Could you check a few things on this drawing? It's one solid part, dimensions in mm from its lowest x, y, z. A direction names the side the tool comes from. Coordinates: 2 decimals unless noted, no trailing zeros. Order: outer loops, then holes, each group sorted by start corner. A loop starts at its lowest first (then second) coordinate and runs counter-clockwise, first axis right, second up. Notation, with made-up numbers: (2.25, -7) - (53.25, -7) arc R18 ccw to (53.25, 6) - close; hole circle Ø10 at (0.5, 0.25). An arc over 180 degrees is marked (long way). Answer in a Markdown table with one row per item. Add a question column.
Item 1: I want a section at C-C (y = 16). Please give me the cut outline in (x, z).
Item 2: Will these pins go through, and if not, where does the flat tip stop? pin 1 Ø12.5 at (x, y) = (27, 18.5) entering from +Z; pin 2 Ø10 at (x, z) = (68, 54) entering from +Y.
Item 3: I want a section at B-B (z = 14). Please give me the cut outline in (x, y).
Item 4: On a 3-axis mill with a long thin cutter (end or side, diameter ignored), from which of +Z, -Z, +X, -X, +Y, -Y can I reach the whole of each face in a straight line? I mean the marked faces 1 and 2. Say none if no direction works.
Item 5: I want a section at A-A (x = 83). Please give me the cut outline in (y, z).
Item 6: If I drill on line 1 along Y through (x, z) = (23.5, 67); line 2 along Z through (x, y) = (48, 1.5), over which ranges is the centre line in solid material (lowest first)? Write a range as from..to.
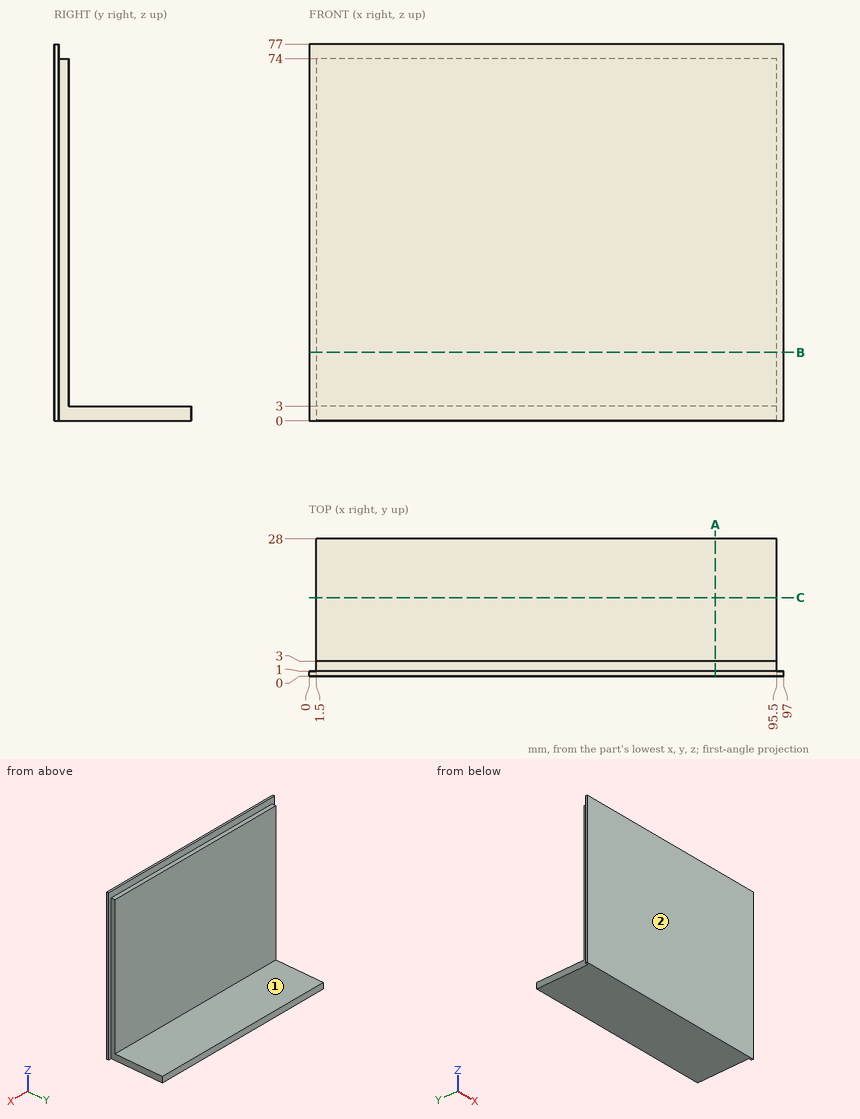
Values follow:
| question | item | result |
|---|---|---|
| 1 | outline | (1.5, 0) - (95.5, 0) - (95.5, 3) - (1.5, 3) - close |
| 2 | pin 1 | stops at z = 3 |
| 2 | pin 2 | stops at y = 3 |
| 3 | outline | (0, 0) - (97, 0) - (97, 1) - (95.5, 1) - (95.5, 3) - (1.5, 3) - (1.5, 1) - (0, 1) - close |
| 4 | face 1 | +Z, +X, -X, +Y |
| 4 | face 2 | +Z, -Z, +X, -X, -Y |
| 5 | outline | (0, 0) - (28, 0) - (28, 3) - (3, 3) - (3, 74) - (1, 74) - (1, 77) - (0, 77) - close |
| 6 | line 1 | y = 0..3 |
| 6 | line 2 | z = 0..74 |
